Check sheet for the modelled part. Datum: model origin and axes. Units: mm. A direction names the side the tool comes from. Give positions to 0.01 mm unless a question says otherwise; leave off trailing zeros. Write each loop counter-clockwise with the first axis right and the second up, starting at its lowest first coordinate (ties: lowest second). Pieces come first, ordered by that corner, then holes. Notation, with made-up numbers: (66.5, 1.25) -> (124.5, 1.25) arc R19 cw to (124.5, 26.25) -> close; hole circle Ø9 at (-17, 24.25). An arc over 180 degrees is marked (long way). Answer as a JSON object with one key per item and string values.
from build123d import *

# Parameters (mm, degrees)
SKETCH1_W           = 19.9
SKETCH1_H           = 22.1
SKETCH1_R           = 1.5748
SKETCH1_R_2         = 0.5
BOSS_EXTRUDE1_DEPTH = 1.6
SKETCH2_R           = 8.2
BOSS_EXTRUDE2_DEPTH = 13.9192
FILLET2_R           = 1.27
SKETCH3_W           = 7.72
SKETCH3_H           = 7.9
BOSS_EXTRUDE3_DEPTH = 9.36


with BuildPart() as part:
    # Sketch1 → Boss-Extrude1 (new body)
    with BuildSketch(Plane.XY):
        Rectangle(SKETCH1_W, SKETCH1_H)
        with Locations((-5.55, 8.49)):
            Circle(SKETCH1_R, mode=Mode.SUBTRACT)
        with Locations((7.41, -8.51)):
            Circle(SKETCH1_R, mode=Mode.SUBTRACT)
        with Locations((-8.75, -9.35)):
            Circle(SKETCH1_R_2, mode=Mode.SUBTRACT)
        with Locations((-8.75, -6.81)):
            Circle(SKETCH1_R_2, mode=Mode.SUBTRACT)
        with Locations((-8.75, -4.27)):
            Circle(SKETCH1_R_2, mode=Mode.SUBTRACT)
        with Locations((-8.75, -1.73)):
            Circle(SKETCH1_R_2, mode=Mode.SUBTRACT)
        with Locations((-8.75, 0.81)):
            Circle(SKETCH1_R_2, mode=Mode.SUBTRACT)
        with Locations((-8.75, 3.35)):
            Circle(SKETCH1_R_2, mode=Mode.SUBTRACT)
        with Locations((-8.75, 5.89)):
            Circle(SKETCH1_R_2, mode=Mode.SUBTRACT)
    extrude(amount=BOSS_EXTRUDE1_DEPTH)

    # Sketch2 → Boss-Extrude2 (add)
    with BuildSketch(Plane(origin=(0, 0, 0), x_dir=(-1, 0, 0), z_dir=(0, 0, -1))):
        with Locations((-0.93, -0.01)):
            Circle(SKETCH2_R)
    extrude(amount=BOSS_EXTRUDE2_DEPTH)

    # Fillet2
    fillet2_edges = [part.edges().sort_by_distance(p)[0] for p in [
        (9.13, -0.01, -13.9192),
    ]]
    fillet(fillet2_edges, radius=FILLET2_R)

    # Sketch3 → Boss-Extrude3 (add)
    with BuildSketch(Plane.XY.offset(1.6)):
        with Locations((-2.83, -5.4)):
            Rectangle(SKETCH3_W, SKETCH3_H)
    extrude(amount=BOSS_EXTRUDE3_DEPTH)


solid = part.part
1. Sectioned sample at B-B, the plane z = -3.25. Enter the section's corners in (x, y).
Determined:
{"outline": "circle Ø16.4 at (0.93, -0.01)"}
2. Scan lines: L1, parallel to Y at x = -1, z = 6.5; L2, parallel to Z at x = -4, y = 7.75; L3, parallel to Z at x = -4.5, y = -6.5. Record each from-to range of solid material in increasing order. Write a range as [from, to].
Determined:
{"L1": "[-9.35, -1.45]", "L2": "[0, 1.6]", "L3": "[0, 10.96]"}
3. Sectioned sample at D-D, the plane z = 2.25. Enter the section's corners in (x, y).
Determined:
{"outline": "(-6.69, -9.35) -> (1.03, -9.35) -> (1.03, -1.45) -> (-6.69, -1.45) -> close"}
4. Mould release check, pull along X, two halves, no side actions. Record for faces 6 (the face through (-8.273, 0.96, 0.789)), 7 (the face through (-6.69, -5, 6)), 8 (the face through (1.03, -5, 6)): released by +X, released by -X, zero draft, split by the parting line, or undercut.
Determined:
{"face 6": "undercut", "face 7": "released by -X", "face 8": "released by +X"}
5. Go/stop test with flat-tipped pins: P1, Ø2.5, axis at y = -5, z = 5, coming from the +X side; P2, Ø10, axis at y = 0, z = -3, coming from the +X side; P3, Ø2, axis at x = 6.5, y = 8.5, coming from the -Z side; P4, Ø6, axis at y = -4.5, z = -10.5, coming from the -X side. Record where each tip stops, or that it passes through.
Determined:
{"P1": "x = 1.03", "P2": "x = 9.95", "P3": "z = 0", "P4": "x = -7.13"}
6. Sectioned sample at A-A, the plane y = -0.01. Enter the section's corners in (x, z).
Determined:
{"outline": "(-9.95, 0) -> (-7.27, 0) -> (-7.27, -12.65) arc R1.27 ccw to (-6, -13.92) -> (7.86, -13.92) arc R1.27 ccw to (9.13, -12.65) -> (9.13, 0) -> (9.95, 0) -> (9.95, 1.6) -> (-9.95, 1.6) -> close"}
7. Access from +Z, -Z, +X, -X, +Y, -Y to the whole of each face (thin tool, end or side, straight path). Record for faces 1 (the face through (-2, 8, 0)), 2 (the face through (-3, -1.45, 6)), 3 (the face through (-3, -9.35, 6)), 4 (the face through (-8.273, 6.04, 0.789)), 5 (the face through (9.95, 0, 1)).
Determined:
{"face 1": "-Z", "face 2": "+Z, +X, -X, +Y", "face 3": "+Z, +X, -X, -Y", "face 4": "+Z, -Z", "face 5": "+Z, -Z, +X, +Y, -Y"}
8. Sectioned sample at C-C, the plane x = -7.75. Enter the section's corners in (y, z), plus the area to 3 significant figures.
Determined:
{"outline": "(-11.05, 0) -> (11.05, 0) -> (11.05, 1.6) -> (-11.05, 1.6) -> close", "area": "35.4 mm^2"}
